Source: CAD feature listing. Evaluate the final solid. Frame: model axes, mm. Face numbers are marked on the shaded views. A direction names the side the tool comes from. Give positions to 0.01 mm unless a question says otherwise; leave off trailing zeros. Loops run counter-clockwise (first coordinate to the right, second up) from the corner with the lowest first, then second, coordinate; pieces in that order, holes last.
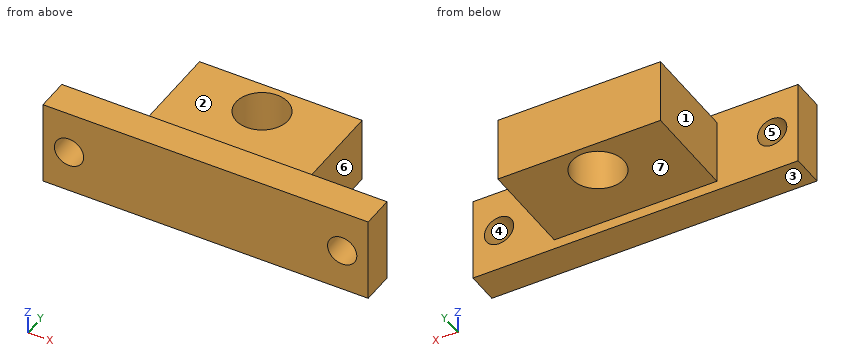
```python
from build123d import *

# Parameters (mm, degrees)
SKETCH1_W           = 50
SKETCH1_H           = 13
BOSS_EXTRUDE1_DEPTH = 5
SKETCH2_R           = 2.25
CUT_EXTRUDE1_DEPTH  = 5
SKETCH3_W           = 25
SKETCH3_H           = 10
BOSS_EXTRUDE2_DEPTH = 15
SKETCH4_R           = 4
CUT_EXTRUDE2_DEPTH  = 15


with BuildPart() as part:
    # Sketch1 → Boss-Extrude1 (new body)
    with BuildSketch(Plane(origin=(0, 0, 0), x_dir=(1, 0, 0), z_dir=(0, 1, 0))):
        Rectangle(SKETCH1_W, SKETCH1_H)
    extrude(amount=BOSS_EXTRUDE1_DEPTH)

    # Sketch2 → Cut-Extrude1 (cut)
    with BuildSketch(Plane(origin=(0, 5, 0), x_dir=(1, 0, 0), z_dir=(0, 1, 0))):
        with Locations(Location((-21, 0, 0), (0, 0, 270))):
            Circle(SKETCH2_R)
        with Locations(Location((21, 0, 0), (0, 0, 270))):
            Circle(SKETCH2_R)
    extrude(amount=-CUT_EXTRUDE1_DEPTH, mode=Mode.SUBTRACT)

    # Sketch3 → Boss-Extrude2 (add)
    with BuildSketch(Plane(origin=(0, 5, 0), x_dir=(1, 0, 0), z_dir=(0, 1, 0))):
        Rectangle(SKETCH3_W, SKETCH3_H)
    extrude(amount=BOSS_EXTRUDE2_DEPTH)

    # Sketch4 → Cut-Extrude2 (cut)
    with BuildSketch(Plane.XY.offset(5)):
        with Locations((0, 15)):
            Circle(SKETCH4_R)
    extrude(amount=-CUT_EXTRUDE2_DEPTH, mode=Mode.SUBTRACT)


solid = part.part
```
(1) Section B-B, the plane y = 15. Return the cut outline in (x, z).
A:
outline: (-12.5, -5) - (-4, -5) - (-4, 5) - (-12.5, 5) - close; (4, -5) - (12.5, -5) - (12.5, 5) - (4, 5) - close
(2) First-contact query: pin 1 (4 mm diameter, centred on y = 9, z = -3.5, fed in from -X); pin 2 (1 mm diameter, centred on y = 9, z = 4.5, fed in from +X); pin 3 (4.5 mm diameter, centred on x = -6, y = 16, fed in from +Z); pin 4 (4 mm diameter, centred on x = -21, z = 0, fed in from +Y). Flat tips, straight axial feed; report the tip coordinate or a pass-through.
A:
pin 1: stops at x = -12.5
pin 2: stops at x = 12.5
pin 3: stops at z = 5
pin 4: passes through
(3) Section C-C, the plane x = 21. Return the cut outline in (y, z), then the cut area to 3 significant figures.
A:
outline: (0, -6.5) - (5, -6.5) - (5, -2.25) - (0, -2.25) - close; (0, 2.25) - (5, 2.25) - (5, 6.5) - (0, 6.5) - close
area: 42.5 mm2
(4) Section A-A, the plane z = 0. Return the cut outline in (x, y).
A:
outline: (-25, 0) - (-23.25, 0) - (-23.25, 5) - (-25, 5) - close; (-18.75, 0) - (18.75, 0) - (18.75, 5) - (12.5, 5) - (12.5, 20) - (-12.5, 20) - (-12.5, 5) - (-18.75, 5) - close; (23.25, 0) - (25, 0) - (25, 5) - (23.25, 5) - close; hole circle Ø8 at (0, 15)
(5) Ray query, line 1 along X through (y, z) = (2.65, 0); line 2 along Y through (x, z) = (0, -2.5); line 3 along Y through (x, z) = (5, -5.5). Return the intervals inside material, ascending.
A:
line 1: x = -25 to -23.25, -18.75 to 18.75, 23.25 to 25
line 2: y = 0 to 11, 19 to 20
line 3: y = 0 to 5
(6) Mould query, pull axis Z, two halves, no side actions, for the marked faces 1, 2, 3 and 4. Classes: pulls with the +Z half, pulls with the -Z half, needs draft (parallel to the pull), parting line crosses it, or undercut.
A:
face 1: needs draft
face 2: pulls with the +Z half
face 3: pulls with the -Z half
face 4: undercut
(7) Section D-D, the plane z = -3.5. Return the cut outline in (x, y).
A:
outline: (-25, 0) - (25, 0) - (25, 5) - (12.5, 5) - (12.5, 20) - (-12.5, 20) - (-12.5, 5) - (-25, 5) - close; hole circle Ø8 at (0, 15)
(8) Reachability of the marked faces 5, 6 and 7 from +Z, -Z, +X, -X, +Y, -Y: full face, straight path, thin tool, end or side. Return the list, or none.
A:
face 5: +Y, -Y
face 6: +Z, -Z, +X, +Y
face 7: -Z, +X, -X, +Y
